Study the drawing (mm; zero at the part's minimum x, y, z) and answer. A direction names the side the tool comes from. Coordinates: 2 decimals unless noted, no trailing zeros. Order: outer loops, then holes, each group sorted by start corner. A loop starts at its lowest first (then second) coordinate and runs counter-clockwise, first axis right, second up.
1. Flat-ended cylindrical pins translate along their axes: pin 1 Ø12 at (x, y) = (28.5, 14.5) entering from -Z; pin 2 Ø10 at (x, y) = (24, 27.5) entering from +Z. Find the tip coordinate at first contact, or state that the pin passes through.
2. Find the intervals of material crossed by probe 1 along Y at (x, z) = (24.5, 2.5); probe 2 along X at (y, z) = (21.5, 4.7); probe 3 along Z at (x, y) = (25.5, 37), in increasing order.
3. The part is cut by section C-C, the plane y = 27.5. Give the vertices of the cut face in (x, z), then the cut area to 3 significant figures.
4. The part is cut by section B-B, the plane x = 12. Give the vertices of the cut face in (y, z), then the cut area to 3 significant figures.
5. The part is cut by section A-A, the plane z = 2.6. Give the vertices of the cut face in (x, y).
6. A tool of negligible diameter and unlimited length cuts with its end or side. For the marked faces 1 and 2, from which of +Z, -Z, +X, -X, +Y, -Y can it reach the whole face along a straight path? Write none if from no direction.
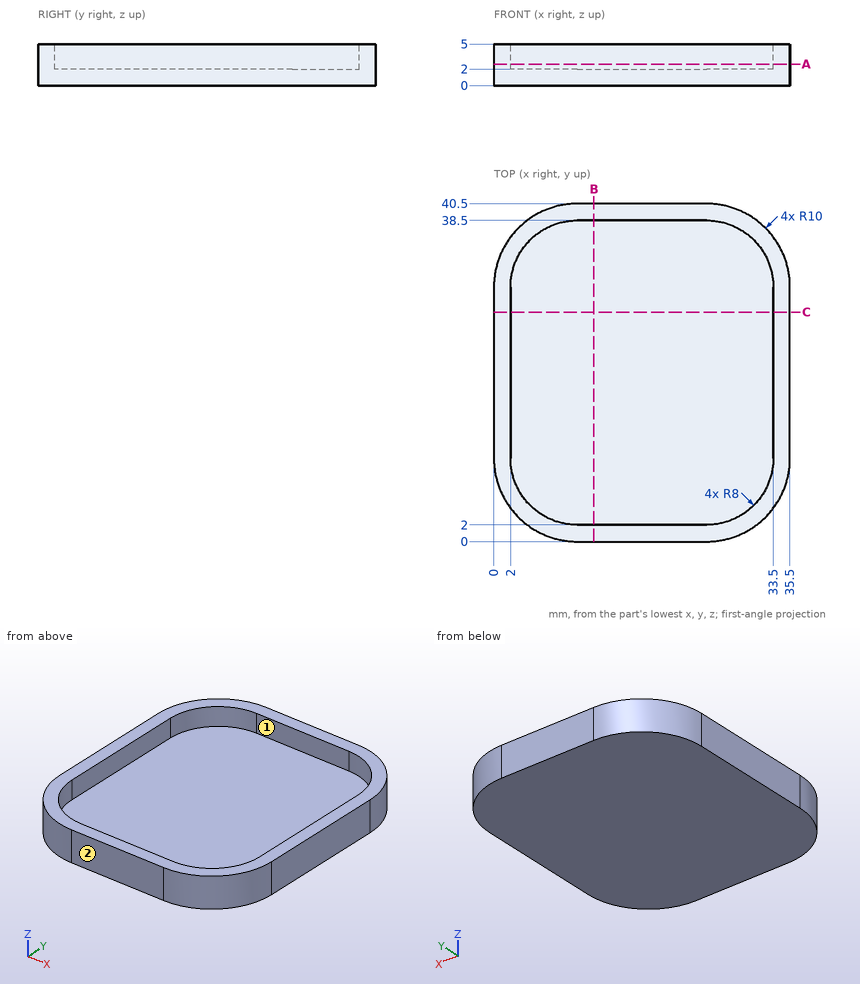
Geometry says:
1. pin 1: stops at z = 0
1. pin 2: stops at z = 2
2. probe 1: y = 0 to 2, 38.5 to 40.5
2. probe 2: x = 0 to 2, 33.5 to 35.5
2. probe 3: z = 0 to 2
3. outline: (0, 0) - (35.5, 0) - (35.5, 5) - (33.5, 5) - (33.5, 2) - (2, 2) - (2, 5) - (0, 5) - close
3. area: 83.0 mm2
4. outline: (0, 0) - (40.5, 0) - (40.5, 5) - (38.5, 5) - (38.5, 2) - (2, 2) - (2, 5) - (0, 5) - close
4. area: 93.0 mm2
5. outline: (0, 10) arc R10 ccw to (10, 0) - (25.5, 0) arc R10 ccw to (35.5, 10) - (35.5, 30.5) arc R10 ccw to (25.5, 40.5) - (10, 40.5) arc R10 ccw to (0, 30.5) - close; hole (2, 10) arc R8 ccw to (10, 2) - (25.5, 2) arc R8 ccw to (33.5, 10) - (33.5, 30.5) arc R8 ccw to (25.5, 38.5) - (10, 38.5) arc R8 ccw to (2, 30.5) - close
6. face 1: +Z
6. face 2: +Z, -Z, +X, -X, -Y
